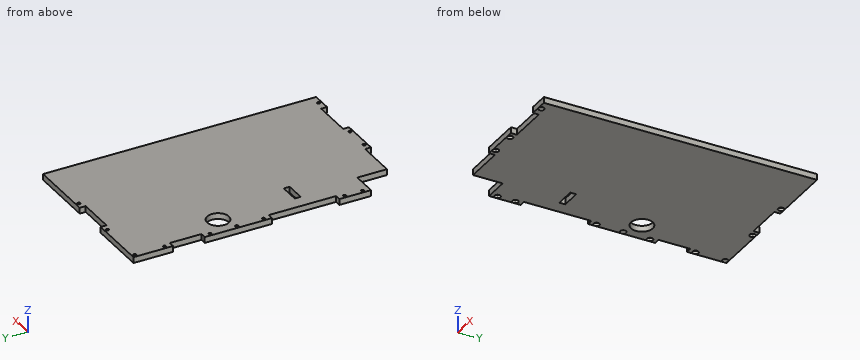
from build123d import *

# Parameters (mm, degrees)
ESQUISSE1_W             = 165
ESQUISSE1_H             = 276
BOSS_EXTRU_1_DEPTH      = 6
ESQUISSE2_W             = 38
ESQUISSE2_H             = 6
ESQUISSE2_W_2           = 6
ESQUISSE2_H_2           = 32
ESQUISSE2_H_3           = 68
ESQUISSE2_W_3           = 40
EXTERIEUR_DEPTH         = 10
ESQUISSE3_R             = 11
ESQUISSE3_W             = 20
ESQUISSE3_H             = 6
ENL_V_MAT_EXTRU_2_DEPTH = 322.616230934
ESQUISSE4_R             = 1.5
ENL_V_MAT_EXTRU_3_DEPTH = 322.616230934
ESQUISSE5_R             = 2.995
ENL_V_MAT_EXTRU_4_DEPTH = 3


with BuildPart() as part:
    # Esquisse1 → Boss.-Extru.1 (new body)
    with BuildSketch(Plane.XY):
        with Locations((-82.5, 138)):
            Rectangle(ESQUISSE1_W, ESQUISSE1_H)
    extrude(amount=BOSS_EXTRU_1_DEPTH)

    # Esquisse2 → exterieur (cut)
    with BuildSketch(Plane.XY.offset(6)):
        with Locations((-86, 273)):
            Rectangle(ESQUISSE2_W, ESQUISSE2_H)
        with Locations((-162, 220)):
            Rectangle(ESQUISSE2_W_2, ESQUISSE2_H_2)
        with Locations((-162, 102)):
            Rectangle(ESQUISSE2_W_2, ESQUISSE2_H_3)
        Polygon((-140, 36), (-140, 6), (-100, 6), (-100, 0), (-165, 0), (-165, 36), align=None)
        with Locations((-40, 3)):
            Rectangle(ESQUISSE2_W_3, ESQUISSE2_H)
    extrude(amount=-EXTERIEUR_DEPTH, mode=Mode.SUBTRACT)

    # Esquisse3 → Enlèv. mat.-Extru.2 (cut, through all)
    with BuildSketch(Plane.XY.offset(6)):
        with Locations((-144, 178.92)):
            Circle(ESQUISSE3_R)
        with Locations((-135, 99)):
            Rectangle(ESQUISSE3_W, ESQUISSE3_H)
    extrude(amount=-ENL_V_MAT_EXTRU_2_DEPTH, mode=Mode.SUBTRACT)

    # Esquisse4 → Enlèv. mat.-Extru.3 (cut, through all)
    with BuildSketch(Plane.XY.offset(6)):
        with Locations((-60, 273)):
            Circle(ESQUISSE4_R)
        with Locations((-112, 273)):
            Circle(ESQUISSE4_R)
        with Locations((-162, 197)):
            Circle(ESQUISSE4_R)
        with Locations((-162, 170)):
            Circle(ESQUISSE4_R)
        with Locations((-162, 143)):
            Circle(ESQUISSE4_R)
        with Locations((-162, 61)):
            Circle(ESQUISSE4_R)
        with Locations((-162, 43)):
            Circle(ESQUISSE4_R)
        with Locations((-93, 3)):
            Circle(ESQUISSE4_R)
        with Locations((-67, 3)):
            Circle(ESQUISSE4_R)
        with Locations((-10, 3)):
            Circle(ESQUISSE4_R)
        with Locations((-162, 273)):
            Circle(ESQUISSE4_R)
        with Locations((-162, 243)):
            Circle(ESQUISSE4_R)
    extrude(amount=-ENL_V_MAT_EXTRU_3_DEPTH, mode=Mode.SUBTRACT)

    # Esquisse5 → Enlèv. mat.-Extru.4 (cut)
    with BuildSketch(Plane(origin=(0, 0, 0), x_dir=(-1, 0, 0), z_dir=(0, 0, -1))):
        with Locations((60, 273)):
            Circle(ESQUISSE5_R)
        with Locations((112, 273)):
            Circle(ESQUISSE5_R)
        with Locations((162, 197)):
            Circle(ESQUISSE5_R)
        with Locations((162, 170)):
            Circle(ESQUISSE5_R)
        with Locations((162, 143)):
            Circle(ESQUISSE5_R)
        with Locations((162, 61)):
            Circle(ESQUISSE5_R)
        with Locations((162, 43)):
            Circle(ESQUISSE5_R)
        with Locations((93, 3)):
            Circle(ESQUISSE5_R)
        with Locations((67, 3)):
            Circle(ESQUISSE5_R)
        with Locations((10, 3)):
            Circle(ESQUISSE5_R)
        with Locations((162, 273)):
            Circle(ESQUISSE5_R)
        with Locations((162, 243)):
            Circle(ESQUISSE5_R)
    extrude(amount=-ENL_V_MAT_EXTRU_4_DEPTH, mode=Mode.SUBTRACT)


solid = part.part
Check sheet for the modelled part. Datum: model origin and axes. Units: mm. Round coordinates to 2 decimals unless told otherwise and drop trailing zeros. Order: outer loops, then holes, each group sorted by start corner. A loop starts at its lowest first (then second) coordinate and runs counter-clockwise, first axis right, second up.
Q1. Scan lines: L1, parallel to X at y = 197, z = 4.3; L2, parallel to Y at x = -24, z = 3.65; L3, parallel to X at y = 82, z = 5.1. Record each from-to range of solid material in increasing order.
Filled sheet:
L1: x = -165 to -163.5, -160.5 to 0
L2: y = 6 to 276
L3: x = -159 to 0
Q2. Depth check by flat-ended pin: P1, Ø3, axis at x = -137, z = 2, coming from the -Y side; P2, Ø5, axis at x = -93, y = 3, coming from the -Z side; P3, Ø2, axis at x = -80, z = 5, coming from the +Y side. Enter the tip coordinate at first touch or a pass-through.
Filled sheet:
P1: stops at y = 6
P2: stops at z = 3
P3: stops at y = 270
Q3. Cross-section at C-C, the plane y = 30. Enter the section's corners in (x, z).
Filled sheet:
outline: (-140, 0) - (0, 0) - (0, 6) - (-140, 6) - close
Q4. Cross-section at A-A, the plane x = -74. Enter the section's corners in (y, z), plus the area to 3 significant figures.
Filled sheet:
outline: (0, 0) - (270, 0) - (270, 6) - (0, 6) - close
area: 1,620 mm2
Q5. Cross-section at B-B, the plane z = 1.5. Give the number of separate pieces and of enclosed holes in the cut face, plus the area to 3 significant figures.
Filled sheet:
separate pieces: 1
enclosed holes: 14
area: 42,500 mm2
